The model under review builds one solid part; all positions refer to its coordinate system, in mm. Face numbers are marked on the shaded views. A direction names the side the tool comes from. Coordinates: 2 decimals unless noted, no trailing zeros. Loops run counter-clockwise (first coordinate to the right, second up) from the corner with the lowest first, then second, coordinate; pieces in that order, holes last. Notation, with made-up numbers: M 74,33.5 L 99,33.5 A30 cw 99,72.5 Z; hole C 88.5,-13 d1. An arc over 180 degrees is marked long. Use CSV: the item, a comma, the result in double quotes. Start each with the question number.
1. Add section C-C, the plane z = 11. Write out the cut boundary in (x, y).
2. Clearance check with flat-ended pins moving along their axes: P1, Ø5, axis at y = -9, z = 9.5, coming from the -X side; P2, Ø1.8, axis at x = -2, z = 2, coming from the +Y side; P3, Ø5, axis at x = -12, z = 4.5, coming from the +Y side. State where each tip first meets the part, or that it passes through.
3. Add section B-B, the plane z = 4.5. Write out the cut boundary in (x, y).
4. Add section A-A, the plane x = 9.5. Write out the cut boundary in (y, z), then the cut area to 3 significant figures.
5. Tool access review of the marked faces 1, 2, 3, 4 and 5: name each direction out of +Z, -Z, +X, -X, +Y, -Y from which nothing blocks a thin tool from reaching the whole face with its end or side.
6. Add section D-D, the plane z = 20. Write out the cut boundary in (x, y), then the cut area to 3 significant figures.
7. Draft analysis for pull direction Y (two halves, no side actions). For the marked faces 6, 7, 8 and 9, state which applies: +Y half, -Y half, draft (parallel to the pull), parting line (faces both ways), or undercut.
8. For L1, parallel to Y at x = 9.5, z = 4.75; L2, parallel to Z at x = 16, y = 7; L3, parallel to Y at x = -3.5, z = 19, list the stretches that pass through material, from the lowest coordinate up.
Autodesk Inventor part; units mm, degrees
ref_plane "YZ Plane" through (0, 0, 0) normal (1, 0, 0) x (0, 1, 0)
ref_plane "XZ Plane" through (0, 0, 0) normal (0, 1, 0) x (-1, 0, 0)
ref_plane "XY Plane" through (0, 0, 0) normal (0, 0, 1) x (1, 0, 0)
sketch "Esboço1" plane through (0, 0, 0) normal (0, 0, 1) x (1, 0, 0)
  line L0 (19.5, -14) -> (19.5, 14)
  line L1 (-19.5, -14) -> (19.5, 14) construction
  line L2 (19.5, -14) -> (-19.5, 14) construction
  circle A0 centre (9.5, 14) radius 10
  circle A1 centre (9.5, 14) radius 5
  line L3 (-19.5, -14) -> (-19.5, -4)
  line L4 (-0.4993, 13.8849) -> (-6.4993, 13.8849)
  line L5 (-19.5, -4) -> (-6.4993, 13.8849)
  line L6 (-19.5, -14) -> (-7, -14)
  line L7 (-7, -14) -> (-7, -4)
  line L8 (-7, -4) -> (8, -4)
  line L9 (8, -4) -> (8, -14)
  line L10 (8, -14) -> (19.5, -14)
  line L11 (-7, -14) -> (8, -14)
  point P0 (0, 0)
  dimension "d0" = 28
  dimension "d2" = 20
  dimension "d3" = 10
  dimension "d5" = 10
  dimension "d6" = 6
  dimension "d8" = 12.5
  dimension "d9" = 15
  dimension "d10" = 10
  dimension "d11" = 10
  dimension "d12" = 15
  dimension "d13" = 11.5
  dimension "d14" = 22.1107
extrude "Extrusão1" add sketch "Esboço1" along normal blind 6
sketch "Esboço2" plane through (0, 0, 6) normal (0, 0, 1) x (1, 0, 0)
  line L0 (-7, -14) -> (-7, -4)
  line L1 (-7, -4) -> (8, -4)
  line L2 (8, -4) -> (8, -14)
  line L3 (-19.5, -4) -> (-19.5, -14)
  line L4 (-19.5, -14) -> (-7, -14)
  line L5 (-7, -14) -> (8, -14)
  line L6 (8, -14) -> (18.5, -14)
  point P0 (0, 0)
  dimension "d17" = 90
  dimension "d18" = 10
  dimension "d19" = 15
  dimension "d20" = 12.5
  dimension "d21" = 10.5
  dimension "d22" = 15
extrude "Extrusão2" add sketch "Esboço2" along normal blind 16
sketch "Esboço3" plane through (-7, -4, 6) normal (0, 1, 0) x (1, 0, 0)
  circle A0 centre (7.4721, -8.5158) radius 4
  point P0 (7, 6)
  dimension "d25" = 8
fillet "Arredondamento1" radius 5 2 edges at (8, -9, 22) (-7, -9, 22)
hole "Furo1" at (0.4721, -4, 14.5158) direction (0, -1, 0) diameter 8 end through all
properties part number "Prova1"
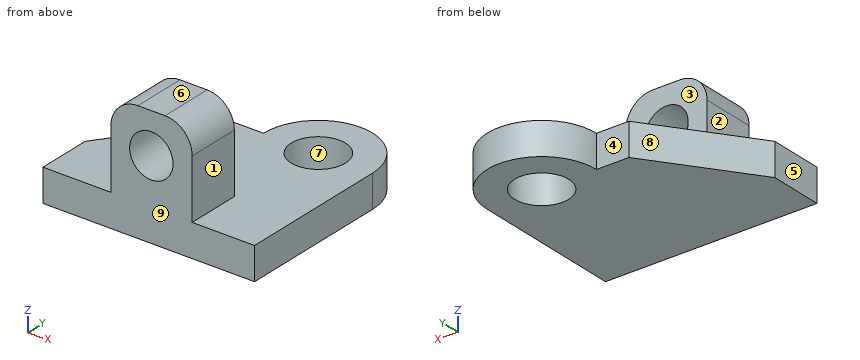
Computed:
1,outline,"M -7,-14 L -1.44,-14 L -1.44,-4 L -7,-4 Z; M 2.38,-14 L 8,-14 L 8,-4 L 2.38,-4 Z"
2,P1,"stops at x = -7"
2,P2,"stops at y = 13.88"
2,P3,"stops at y = 9.76"
3,outline,"M -19.5,-14 L 19.5,-14 L 19.5,14 A10 ccw long -0.5,13.88 L -6.5,13.88 L -19.5,-4 Z; hole C 9.5,14 d10"
4,outline,"M -14,0 L 9,0 L 9,6 L -14,6 Z; M 19,0 L 24,0 L 24,6 L 19,6 Z"
4,area,"168 mm^2"
5,face 1,"+Z, +X, +Y, -Y"
5,face 2,"+Z, -X, +Y, -Y"
5,face 3,"+Z, +X, -X, +Y"
5,face 4,"+Z, -Z, -X, +Y"
5,face 5,"+Z, -Z, -X, +Y, -Y"
6,outline,"M -6,-14 L 7,-14 L 7,-4 L -6,-4 Z"
6,area,"130 mm^2"
7,face 6,"draft"
7,face 7,"undercut"
7,face 8,"+Y half"
7,face 9,"-Y half"
8,L1,"y = -14 to 9, 19 to 24"
8,L2,"z = 0 to 6"
8,L3,"y = -14 to -4"
